from build123d import *

# Parameters (mm, degrees)
SKETCH1_R           = 75
BOSS_EXTRUDE1_DEPTH = 10
SKETCH2_R           = 19
BOSS_EXTRUDE2_DEPTH = 30
SKETCH3_R           = 11
CUT_EXTRUDE1_DEPTH  = 114.357840488
SKETCH5_R           = 25
CUT_EXTRUDE2_DEPTH  = 113.269764407
CIRPATTERN1_COUNT   = 4
SKETCH6_R           = 10
CUT_EXTRUDE3_DEPTH  = 113.269764407
CIRPATTERN2_COUNT   = 4


with BuildPart() as part:
    # Sketch1 → Boss-Extrude1 (new body)
    with BuildSketch(Plane.XY):
        Circle(SKETCH1_R)
    extrude(amount=BOSS_EXTRUDE1_DEPTH)

    # Sketch2 → Boss-Extrude2 (add)
    with BuildSketch(Plane.XY.offset(10)):
        Circle(SKETCH2_R)
    extrude(amount=BOSS_EXTRUDE2_DEPTH)

    # Sketch3 → Cut-Extrude1 (cut, through all)
    with BuildSketch(Plane.XY.offset(40)):
        Circle(SKETCH3_R)
    extrude(amount=-CUT_EXTRUDE1_DEPTH, mode=Mode.SUBTRACT)

    # Sketch4 → Revolve1 (revolve)
    with BuildSketch(Plane(origin=(0, 0, 0), x_dir=(1, 0, 0), z_dir=(0, 1, 0))):
        Polygon((75, 0), (76.5, 0), (75, -2), align=None)
        Polygon((75, -10), (76.5, -10), (75, -8), align=None)
    revolve(axis=Axis((0, 0, 40), (0, 0, -1)))

    # Sketch5 → Cut-Extrude2 (cut, through all)
    with BuildSketch(Plane.XY.offset(10)):
        with Locations((0, 45)):
            Circle(SKETCH5_R)
    cut_extrude2 = extrude(amount=-CUT_EXTRUDE2_DEPTH, mode=Mode.SUBTRACT)

    # CirPattern1: Cut-Extrude2 ×4 about axis
    cirpattern1_axis = Axis((0, 0, 0), (0, 0, 1))
    for i in range(1, CIRPATTERN1_COUNT):
        add(cut_extrude2.rotate(cirpattern1_axis, i * 360 / CIRPATTERN1_COUNT), mode=Mode.SUBTRACT)

    # Sketch6 → Cut-Extrude3 (cut, through all)
    with BuildSketch(Plane.XY.offset(10)):
        with Locations((38.890872965, 38.890872965)):
            Circle(SKETCH6_R)
    cut_extrude3 = extrude(amount=-CUT_EXTRUDE3_DEPTH, mode=Mode.SUBTRACT)

    # CirPattern2: Cut-Extrude3 ×4 about axis
    cirpattern2_axis = Axis((0, 0, 0), (0, 0, 1))
    for i in range(1, CIRPATTERN2_COUNT):
        add(cut_extrude3.rotate(cirpattern2_axis, i * 360 / CIRPATTERN2_COUNT), mode=Mode.SUBTRACT)


solid = part.part
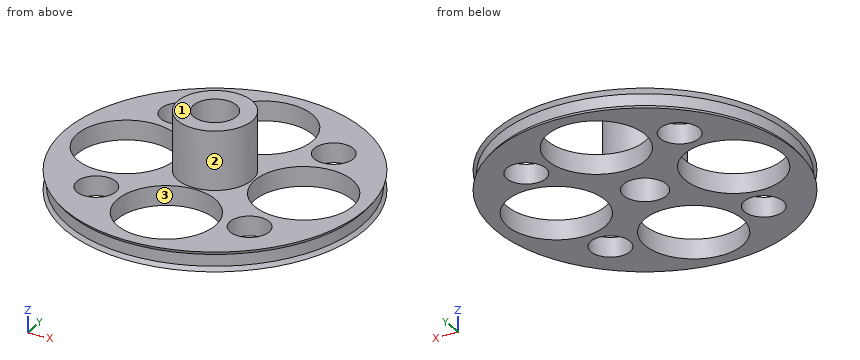
Input: part model. Units: mm. Frame: model coordinates. Face numbers are marked on the shaded views. Give positions to 0.01 mm unless a question says otherwise; leave off trailing zeros. Write each loop counter-clockwise with the first axis right and the second up, starting at its lowest first coordinate (ties: lowest second). Pieces come first, ordered by that corner, then holes. Notation, with made-up numbers: M 41.25,11 L 79.25,11 A16 cw 79.25,25 Z; hole C 67.5,-32 d7. An arc over 180 degrees is marked long. Use one line per item in the form item = value.
1. Cut plane C-C on y = -45. State how many separate pieces and enclosed holes the cut face has, and give its area (3 significant figures).
Outcome:
separate_pieces = 4
enclosed_holes = 0
area = 391 mm²
2. Cut plane A-A on x = 0. Return loops of the section in (y, z).
Outcome:
outline = M -76.5,0 L -70,0 L -70,10 L -76.5,10 L -75,8 L -75,2 Z; M -20,0 L -11,0 L -11,40 L -19,40 L -19,10 L -20,10 Z; M 11,0 L 20,0 L 20,10 L 19,10 L 19,40 L 11,40 Z; M 70,0 L 76.5,0 L 75,2 L 75,8 L 76.5,10 L 70,10 Z
3. Cut plane B-B on z = 22. Return loops of the section in (x, y).
Outcome:
outline = C 0,0 d38; hole C 0,0 d22
4. Ray query, L1, parallel to Y at x = 0, z = 4; L2, parallel to X at y = 22, z = 2; L3, parallel to X at y = 8, z = 2. Return the intervals inside material, ascending.
Outcome:
L1 = -75 to -70, -20 to -11, 11 to 20, 70 to 75
L2 = -71.7 to -56.87, -33.13 to -9.8, 9.8 to 33.13, 56.87 to 71.7
L3 = -74.57 to -68.69, -21.31 to -7.55, 7.55 to 21.31, 68.69 to 74.57
5. Mould query, pull axis Y, two halves, no side actions, for the marked faces 1, 2 and 3. Classes: released by +Y, released by -Y, zero draft, split by the parting line, or undercut.
Outcome:
face_1 = zero draft
face_2 = split by the parting line
face_3 = undercut
6. First-contact query: P1, Ø10, axis at x = 3, z = 26, coming from the +Y side; P2, Ø3, axis at x = -45.5, y = 29.5, coming from the -Z side; P3, Ø8, axis at x = 60.5, y = 52.5, coming from the +Z side. Flat tips, straight axial feed; report the tip coordinate or a pass-through.
Outcome:
P1 = 19
P2 = 0
P3 = 10
